from build123d import *

# Parameters (mm, degrees)
F0_R     = 6
F0_R_2   = 4
F1_DEPTH = 13
F0_R_3   = 3
F2_DEPTH = 12
F3_SIZE  = 0.99999
F4_SIZE  = 0.5


# Not quite as in the source:
# - a fillet or chamfer is up to 0.001 mm smaller than in the source, because OpenCascade refuses the exact size


with BuildPart() as f1:
    # F0 (on Top) → F1 (new body)
    with BuildSketch(Plane.XY):
        Circle(F0_R)
        Circle(F0_R_2, mode=Mode.SUBTRACT)
    extrude(amount=-F1_DEPTH)

    # F0 (on Top) → F2 (join)
    with BuildSketch(Plane.XY):
        Circle(F0_R)
        Circle(F0_R_2, mode=Mode.SUBTRACT)
        Circle(F0_R_2)
        Circle(F0_R_3, mode=Mode.SUBTRACT)
    extrude(amount=F2_DEPTH)

    # F3 (size 1 in the source; OpenCascade refuses exactly that, so slightly less here)
    f3_edges = [f1.edges().sort_by_distance(p)[0] for p in [
        (-3, 0, 0),
    ]]
    chamfer(f3_edges, length=F3_SIZE)

    # F4
    f4_edges = [f1.edges().sort_by_distance(p)[0] for p in [
        (-4, 0, -13),
    ]]
    chamfer(f4_edges, length=F4_SIZE)


solid = f1.part
Here's how the part is built. I have some questions about the finished solid (model axes, mm). Round coordinates to 2 decimals unless told otherwise and drop trailing zeros. Order: outer loops, then holes, each group sorted by start corner. A loop starts at its lowest first (then second) coordinate and runs counter-clockwise, first axis right, second up. Notation, with made-up numbers: (81.5, 58.25) -> (134.5, 58.25) arc R28 ccw to (134.5, 84.25) -> close; hole circle Ø8 at (34.25, 3). An arc over 180 degrees is marked (long way). Return JSON: item names as keys, results as strings.
Q1. If we mould it in two halves opening along Y, with no side actions, what happens to faces 1 (the cylindrical face through (-0.867, -3.905, -6.162)), 2 (the cylindrical face through (-6, 0, 0)), 3 (the flat face through (-3, -1, 12))? For each: released by +Y, released by -Y, zero draft, split by the parting line, or undercut.
Filled sheet:
{"face 1": "undercut", "face 2": "split by the parting line", "face 3": "zero draft"}
Q2. For pin 1 Ø2.5 at (x, y) = (-1.5, 1.5) entering from -Z; pin 2 Ø1 at (y, z) = (-2, 1) entering from -X; pin 3 Ø5 at (x, y) = (1.5, -1) entering from -Z; pin 4 Ø3.5 at (x, y) = (0, 0) entering from +Z, each with a flat end and sliding along its axis, tell me the tip position at first contact or that it passes through.
Filled sheet:
{"pin 1": "stops at z = 0.63", "pin 2": "stops at x = -5.81", "pin 3": "stops at z = -12.8", "pin 4": "passes through"}
Q3. I need wall thicknesses on line 1 along Y through (x, z) = (0, -9.75); line 2 along Y through (x, z) = (0, 4); line 3 along X through (y, z) = (3.5, -4). Which ranges of each line are inside material? Lowest first, please. Write a range as from..to.
Filled sheet:
{"line 1": "y = -6..-4, 4..6", "line 2": "y = -6..-3, 3..6", "line 3": "x = -4.87..-1.94, 1.94..4.87"}
Q4. If we section it at C-C on z = -8: List the corners of the cut face in (x, y) for me, plus the area to 3 significant figures.
Filled sheet:
{"outline": "circle Ø12 at (0, 0); hole circle Ø8 at (0, 0)", "area": "62.8 mm^2"}
Q5. If we section it at D-D on y = -4.75: List the corners of the cut face in (x, z) for me.
Filled sheet:
{"outline": "(-3.67, -13) -> (3.67, -13) -> (3.67, 12) -> (-3.67, 12) -> close"}
